Can you work these out from the model? Positions are in its coordinate system, mm. A direction names the side the tool comes from. Coordinates: 2 decimals unless noted, no trailing zeros. Loops run counter-clockwise (first coordinate to the right, second up) from the corner with the lowest first, then second, coordinate; pieces in that order, holes last. Notation, with made-up numbers: (86.5, -40) -> (133.5, -40) arc R19 cw to (133.5, -20) -> close; hole circle Ø6 at (8.25, -5). An arc over 180 degrees is marked (long way). Put each result on its own line as item: value. Start each with the question number.
Item 1: For faces 5 (the flat face through (-27.5, 5, 130)), 6 (the flat face through (0, 5, -115)), 7 (the flat face through (-57, 5, 145)), which set-ups out of +Z, -Z, +X, -X, +Y, -Y let a thin tool reach every point of the face, with its end or its side?
Item 2: If we section it at C-C on x = 98: Please give me the cut outline in (y, z), plus the area to 3 significant figures.
Item 3: Will these pins go through, and if not, where does the flat tip stop? P1, Ø5, axis at x = -16, y = 3.5, coming from the +Z side; P2, Ø3, axis at y = 7, z = 132, coming from the +X side; P3, Ø3, axis at y = 7, z = -127, coming from the -X side.
Item 4: If we section it at B-B on y = 7.75: Please give me the cut outline in (x, z).
Item 5: If we section it at A-A on z = -121.5: Please give me the cut outline in (x, y).
Item 6: If we section it at D-D on z = 125: Please give me the cut outline in (x, y).
Item 7: We'd pull the mould along X, two halves only. Please class faces 1 (the flat face through (0, 5, 115)), 2 (the flat face through (100.21, 5.07, 115.85)), 3 (the flat face through (56, 5, -145)), 4 (the flat face through (27.5, 5, 130)): pulls with the +X half, pulls with the -X half, needs draft (parallel to the pull), parting line crosses it, or undercut.
Item 8: Please list where these lines run through material, in increasing order: L1, parallel to Z at x = -8, y = 2.5; L2, parallel to X at y = 4.5, z = 120. Write a range as from..to.
```python
from build123d import *

# Parameters (mm, degrees)
SKETCH1_W           = 310
SKETCH1_H           = 290
BOSS_EXTRUDE1_DEPTH = 10
CUT_EXTRUDE1_DEPTH  = 213.485293609
SKETCH3_W           = 55
SKETCH3_H           = 30
CUT_EXTRUDE2_DEPTH  = 186.33752993


with BuildPart() as part:
    # Sketch1 → Boss-Extrude1 (new body)
    with BuildSketch(Plane(origin=(0, 0, 0), x_dir=(1, 0, 0), z_dir=(0, 1, 0))):
        Rectangle(SKETCH1_W, SKETCH1_H)
    extrude(amount=BOSS_EXTRUDE1_DEPTH)

    # Sketch2 → Cut-Extrude1 (cut, through all)
    with BuildSketch(Plane(origin=(0, 10, 0), x_dir=(1, 0, 0), z_dir=(0, 1, 0))):
        Polygon((-85, 145), (-115.000000002, 87.5), (-115.000000002, -87.5), (-85, -145), (-155, -145), (-155, 145), align=None)
        Polygon((155, -145), (155, 145), (85, 145), (115.000000002, 87.5), (115.000000002, -87.5), (85, -145), align=None)
    extrude(amount=-CUT_EXTRUDE1_DEPTH, mode=Mode.SUBTRACT)

    # Sketch3 → Cut-Extrude2 (cut, through all)
    with BuildSketch(Plane(origin=(0, 10, 0), x_dir=(1, 0, 0), z_dir=(0, 1, 0))):
        with Locations((0, 130)):
            Rectangle(SKETCH3_W, SKETCH3_H)
        with Locations((0, -130)):
            Rectangle(SKETCH3_W, SKETCH3_H)
    extrude(amount=-CUT_EXTRUDE2_DEPTH, mode=Mode.SUBTRACT)


solid = part.part
```
Solutions:
1. face 5: +Z, +Y, -Y
1. face 6: -Z, +Y, -Y
1. face 7: +Z, +X, -X, +Y, -Y
2. outline: (0, -120.08) -> (10, -120.08) -> (10, 120.08) -> (0, 120.08) -> close
2. area: 2,400 mm^2
3. P1: z = 115
3. P2: x = 92.57
3. P3: x = -95.17
4. outline: (-115, -87.5) -> (-85, -145) -> (-27.5, -145) -> (-27.5, -115) -> (27.5, -115) -> (27.5, -145) -> (85, -145) -> (115, -87.5) -> (115, 87.5) -> (85, 145) -> (27.5, 145) -> (27.5, 115) -> (-27.5, 115) -> (-27.5, 145) -> (-85, 145) -> (-115, 87.5) -> close
5. outline: (-97.26, 0) -> (-27.5, 0) -> (-27.5, 10) -> (-97.26, 10) -> close; (27.5, 0) -> (97.26, 0) -> (97.26, 10) -> (27.5, 10) -> close
6. outline: (-95.43, 0) -> (-27.5, 0) -> (-27.5, 10) -> (-95.43, 10) -> close; (27.5, 0) -> (95.43, 0) -> (95.43, 10) -> (27.5, 10) -> close
7. face 1: undercut
7. face 2: pulls with the +X half
7. face 3: needs draft
7. face 4: undercut
8. L1: -115..115
8. L2: -98.04..-27.5, 27.5..98.04
